Work out the finished part from the listing and answer in its coordinate system (mm). A direction names the side the tool comes from. Round coordinates to 2 decimals unless told otherwise and drop trailing zeros. Order: outer loops, then holes, each group sorted by start corner. A loop starts at its lowest first (then second) coordinate and runs counter-clockwise, first axis right, second up. Notation, with made-up numbers: M 45.5,83 L 59.5,83 A15 cw 59.5,94 Z; hole C -23,0.5 d1. An arc over 180 degrees is marked long. Return JSON: item names as keys, results as strings.
from build123d import *

# Parameters (mm, degrees)
BOSS_EXTRUDE1_DEPTH = 5
SKETCH2_W           = 5
SKETCH2_H           = 62.45
BOSS_EXTRUDE2_DEPTH = 67.45
SKETCH6_R           = 3.25
CUT_EXTRUDE4_DEPTH  = 5
CUT_EXTRUDE5_DEPTH  = 2.1
CUT_EXTRUDE6_DEPTH  = 5
SKETCH8_W           = 15.15
SKETCH8_H           = 5
BOSS_EXTRUDE3_DEPTH = 62.45
SKETCH9_W           = 62.45
SKETCH9_H           = 55
BOSS_EXTRUDE4_DEPTH = 6
SKETCH10_W          = 62.45
SKETCH10_H          = 55
BOSS_EXTRUDE5_DEPTH = 5
BOSS_EXTRUDE6_DEPTH = 6
CUT_EXTRUDE7_DEPTH  = 6
BOSS_EXTRUDE7_DEPTH = 5
SKETCH14_R          = 7.5
CUT_EXTRUDE8_DEPTH  = 5
SKETCH12_3_R        = 1.75
CUT_EXTRUDE9_DEPTH  = 6
SKETCH16_R          = 3
BOSS_EXTRUDE8_DEPTH = 17


with BuildPart() as part:
    # Sketch1 → Boss-Extrude1 (new body)
    with BuildSketch(Plane(origin=(0, 0, 0), x_dir=(1, 0, 0), z_dir=(0, 1, 0))):
        Polygon((-27.5, 0), (-27.5, 31.225), (27.5, 31.225), (27.5, -31.225), (-27.5, -31.225), align=None)
    extrude(amount=-BOSS_EXTRUDE1_DEPTH)

    # Sketch2 → Boss-Extrude2 (add)
    with BuildSketch(Plane.XZ.offset(5)):
        with Locations((30, 0)):
            Rectangle(SKETCH2_W, SKETCH2_H)
        with Locations((-30, 0)):
            Rectangle(SKETCH2_W, SKETCH2_H)
    extrude(amount=-BOSS_EXTRUDE2_DEPTH)

    # Sketch6 → Cut-Extrude4 (cut)
    with BuildSketch(Plane.ZY.offset(-27.5)):
        with Locations((-23.175, 51.4)):
            Circle(SKETCH6_R)
        with Locations((23.175, 5.05)):
            Circle(SKETCH6_R)
    extrude(amount=-CUT_EXTRUDE4_DEPTH, mode=Mode.SUBTRACT)

    # Sketch7 → Cut-Extrude5 (cut)
    with BuildSketch(Plane.ZY.offset(-27.5)):
        with BuildLine():
            Line((0, 47.3), (31.225, 47.3))
            Line((31.225, 47.3), (31.225, 9.15))
            Line((31.225, 9.15), (0, 9.15))
            ThreePointArc((0, 9.15), (-19.075, 28.225), (0, 47.3))
        make_face()
    extrude(amount=-CUT_EXTRUDE5_DEPTH, mode=Mode.SUBTRACT)

    # Sketch7<3> → Cut-Extrude6 (cut)
    with BuildSketch(Plane.ZY.offset(-27.5)):
        with BuildLine():
            Line((0, 32.475), (31.225, 32.475))
            Line((31.225, 32.475), (31.225, 23.975))
            Line((31.225, 23.975), (0, 23.975))
            ThreePointArc((0, 23.975), (-4.25, 28.225), (0, 32.475))
        make_face()
    extrude(amount=-CUT_EXTRUDE6_DEPTH, mode=Mode.SUBTRACT)

    # Sketch8 → Boss-Extrude3 (add)
    with BuildSketch(Plane(origin=(0, 0, -31.225), x_dir=(-1, 0, 0), z_dir=(0, 0, -1))):
        with Locations((35.075, 59.95)):
            Rectangle(SKETCH8_W, SKETCH8_H)
        with Locations((-35.075, 59.95)):
            Rectangle(SKETCH8_W, SKETCH8_H)
    extrude(amount=-BOSS_EXTRUDE3_DEPTH)

    # Sketch9 → Boss-Extrude4 (add)
    with BuildSketch(Plane.ZY.offset(42.65)):
        with Locations((0, 84.95)):
            Rectangle(SKETCH9_W, SKETCH9_H)
    extrude(amount=BOSS_EXTRUDE4_DEPTH)

    # Sketch10 → Boss-Extrude5 (add)
    with BuildSketch(Plane(origin=(42.65, 0, 0), x_dir=(0, 0, -1), z_dir=(1, 0, 0))):
        with Locations((0, 84.95)):
            Rectangle(SKETCH10_W, SKETCH10_H)
    extrude(amount=BOSS_EXTRUDE5_DEPTH)

    # Sketch11 → Boss-Extrude6 (add)
    with BuildSketch(Plane(origin=(-42.65, 0, 0), x_dir=(0, 0, -1), z_dir=(1, 0, 0))):
        with BuildLine():
            Line((-31.225, 112.45), (31.225, 112.45))
            ThreePointArc((31.225, 112.45), (0, 143.675), (-31.225, 112.45))
        make_face()
    extrude(amount=-BOSS_EXTRUDE6_DEPTH)

    # Sketch12 → Cut-Extrude7 (cut)
    with BuildSketch(Plane(origin=(-42.65, 0, 0), x_dir=(0, 0, -1), z_dir=(1, 0, 0))):
        Polygon((7, 112.45), (3.5, 118.512177826), (-3.5, 118.512177826), (-7, 112.45), (-3.5, 106.387822174), (3.5, 106.387822174), align=None)
    extrude(amount=-CUT_EXTRUDE7_DEPTH, mode=Mode.SUBTRACT)

    # Sketch13 → Boss-Extrude7 (add)
    with BuildSketch(Plane.ZY.offset(-42.65)):
        with BuildLine():
            Line((-31.225, 112.45), (31.225, 112.45))
            ThreePointArc((31.225, 112.45), (0, 143.675), (-31.225, 112.45))
        make_face()
    extrude(amount=-BOSS_EXTRUDE7_DEPTH)

    # Sketch14 → Cut-Extrude8 (cut)
    with BuildSketch(Plane.ZY.offset(-42.65)):
        with Locations((0, 112.45)):
            Circle(SKETCH14_R)
    extrude(amount=-CUT_EXTRUDE8_DEPTH, mode=Mode.SUBTRACT)

    # Sketch12<3> → Cut-Extrude9 (cut)
    with BuildSketch(Plane(origin=(-42.65, 0, 0), x_dir=(0, 0, -1), z_dir=(1, 0, 0))):
        with Locations((0, 124.95)):
            Circle(SKETCH12_3_R)
        with Locations((-12.5, 112.45)):
            Circle(SKETCH12_3_R)
        with Locations((0, 99.95)):
            Circle(SKETCH12_3_R)
        with Locations((12.5, 112.45)):
            Circle(SKETCH12_3_R)
    extrude(amount=-CUT_EXTRUDE9_DEPTH, mode=Mode.SUBTRACT)

    # Sketch16 → Boss-Extrude8 (add)
    with BuildSketch(Plane(origin=(-27.5, 0, 0), x_dir=(0, 0, -1), z_dir=(1, 0, 0))):
        with Locations((0, 28.22)):
            Circle(SKETCH16_R)
    extrude(amount=-BOSS_EXTRUDE8_DEPTH)


solid = part.part
Item 1: Find section A-A (y = 99.95). Determine the outline of the cut face in (x, z) (3 decimals).
Output:
{"outline": "M -48.65,-31.225 L -42.65,-31.225 L -42.65,-1.75 L -48.65,-1.75 Z; M -48.65,1.75 L -42.65,1.75 L -42.65,31.225 L -48.65,31.225 Z; M 42.65,-31.225 L 47.65,-31.225 L 47.65,31.225 L 42.65,31.225 Z"}
Item 2: Each of these flat-tipped pins is pushed along its axis until it touches: pin 1 (1.5 mm diameter, centred on y = 19, z = 24.5, fed in from +X); pin 2 (13 mm diameter, centred on x = -39.5, z = -5, fed in from -Y); pin 3 (6 mm diameter, centred on x = -27.5, z = -2, fed in from +Y). Where does it stop, or does it pass through?
Output:
{"pin 1": "stops at x = 32.5", "pin 2": "stops at y = 25.22", "pin 3": "stops at y = 62.45"}
Item 3: Find section B-B (y = 28.22). Determine the outline of the cut face in (x, z) (3 decimals), plus the area to 3 significant figures.
Output:
{"outline": "M -44.5,-3 L -32.5,-3 L -32.5,-31.225 L -27.5,-31.225 L -27.5,31.225 L -32.5,31.225 L -32.5,3 L -44.5,3 Z; M 27.5,-31.225 L 32.5,-31.225 L 32.5,-4.25 L 29.6,-4.25 L 29.6,-19.075 L 27.5,-19.075 Z", "area": "488 mm^2"}
Item 4: The mould has two halves that part along Z. Classify faces 1 (the flat face through (-27.5, 32, 0)), 2 (the cylindrical face through (29.965, 53.597, -25.57)), 3 (the flat face through (28, 45, -31.225)): pulls with the +Z half, pulls with the -Z half, needs draft (parallel to the pull), parting line crosses it, or undercut.
Output:
{"face 1": "needs draft", "face 2": "undercut", "face 3": "pulls with the -Z half"}
Item 5: Which of the six approach directions +Z, -Z, +X, -X, +Y, -Y give full straight-line access (tool end or side, diameter ignored) to faces 4 (the flat face through (32.5, 26, -7)), 5 (the flat face through (-35, 62.45, 0)), 6 (the flat face through (29.6, 33, 6)), 7 (the flat face through (-46, 118.512, 0))?
Output:
{"face 4": "+Z, -Z, +X, -Y", "face 5": "+Z, -Z, +Y", "face 6": "+Z", "face 7": "+X, -X"}
Item 6: Consider line 1 along Y through (x, z) = (-44.05, 0) (3 decimals); line 2 along Y through (x, z) = (-46, 0) (3 decimals); line 3 along X through (y, z) = (115, 26). Determine where each line is inside the solid, lowest interval first. Write a range as [from, to].
Output:
{"line 1": "y = [25.22, 31.22], [57.45, 98.2], [101.7, 106.388], [118.512, 123.2], [126.7, 143.675]", "line 2": "y = [57.45, 98.2], [101.7, 106.388], [118.512, 123.2], [126.7, 143.675]", "line 3": "x = [-48.65, -42.65], [42.65, 47.65]"}
Item 7: Find section C-C (y = 51.4). Determine the outline of the cut face in (x, z) (3 decimals), plus the area to 3 significant figures.
Output:
{"outline": "M -32.5,-31.225 L -27.5,-31.225 L -27.5,31.225 L -32.5,31.225 Z; M 27.5,-31.225 L 32.5,-31.225 L 32.5,-26.425 L 27.5,-26.425 Z; M 27.5,-19.925 L 32.5,-19.925 L 32.5,31.225 L 27.5,31.225 Z", "area": "592 mm^2"}
Item 8: Find section D-D (x = -15). Determine the outline of the cut face in (y, z) (3 decimals).
Output:
{"outline": "M -5,-31.225 L 0,-31.225 L 0,31.225 L -5,31.225 Z"}
